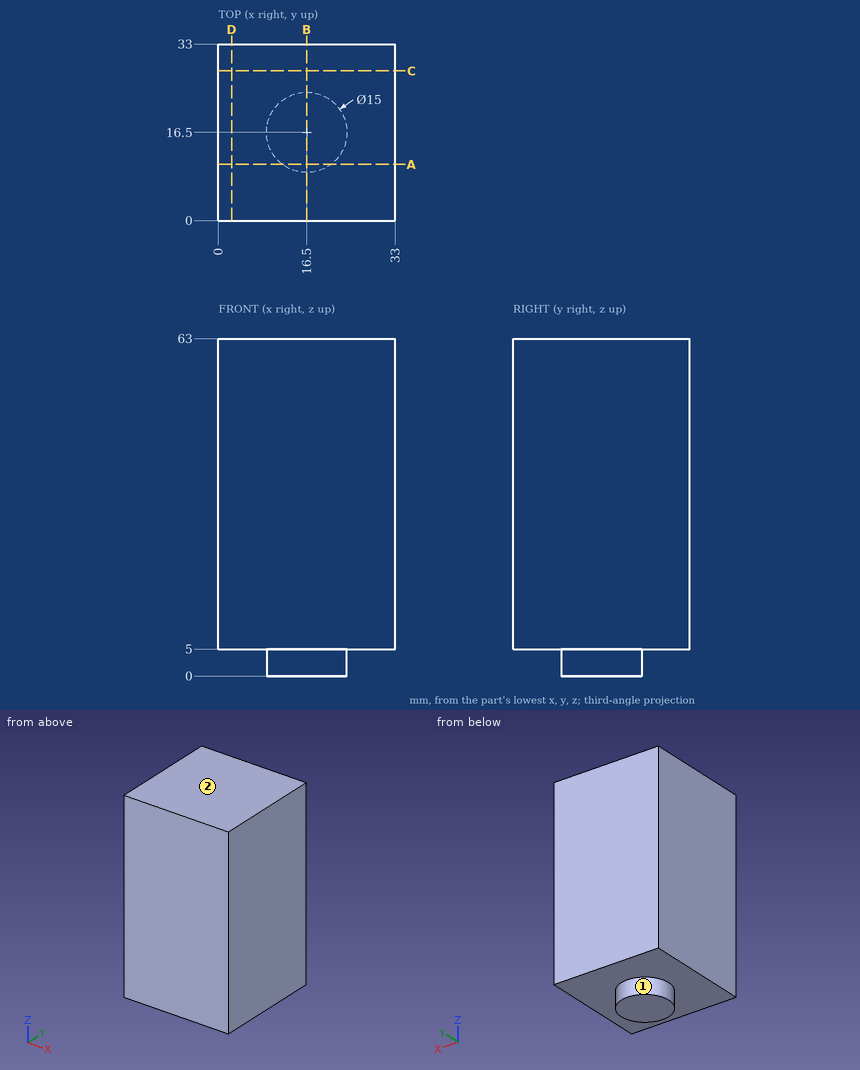
Verification items for this drawing (mm, ordinates from the low corner). A direction names the side the tool comes from. Round coordinates to 2 decimals unless told otherwise and drop trailing zeros. Write each loop counter-clockwise with the first axis right and the second up, starting at its lowest first coordinate (ties: lowest second). Pieces come first, ordered by that corner, then holes. Notation, with made-up numbers: (-6, -25.5) - (36, -25.5) arc R9 ccw to (36, -13.5) - close; hole circle Ø8 at (-8.75, 88.25). An arc over 180 degrees is marked (long way). One line per item, written item: value.
1. Cross-section at A-A on y = 10.5. Record the boundary of the cut face in (x, z).
The answers:
outline: (0, 5) - (12, 5) - (12, 0) - (21, 0) - (21, 5) - (33, 5) - (33, 63) - (0, 63) - close
2. Scan line: L1, parallel to Z at x = 5, y = 27. Record every from-to range of solid material in increasing order.
The answers:
L1: z = 5 to 63
3. Cross-section at B-B on x = 16.5. Record the boundary of the cut face in (y, z), and give its area (3 significant figures).
The answers:
outline: (0, 5) - (9, 5) - (9, 0) - (24, 0) - (24, 5) - (33, 5) - (33, 63) - (0, 63) - close
area: 1,990 mm^2
4. Depth check by flat-ended pin: pin 1 Ø3 at (x, y) = (28.5, 25.5) entering from -Z. Enter the tip coordinate at first touch or a pass-through.
The answers:
pin 1: stops at z = 5
5. Set-up check for the marked faces 1 and 2: record each of +Z, -Z, +X, -X, +Y, -Y from which the full face is reachable in a straight line by a thin tool's end or side.
The answers:
face 1: -Z
face 2: +Z, +X, -X, +Y, -Y
6. Cross-section at C-C on y = 28. Record the boundary of the cut face in (x, z).
The answers:
outline: (0, 5) - (33, 5) - (33, 63) - (0, 63) - close
